Source: CAD feature listing. Evaluate the final solid. Frame: model axes, mm. Face numbers are marked on the shaded views. A direction names the side the tool comes from. Give positions to 0.01 mm unless a question says otherwise; leave off trailing zeros. Loops run counter-clockwise (first coordinate to the right, second up) from the corner with the lowest first, then second, coordinate; pieces in that order, holes last.
from build123d import *

# Parameters (mm, degrees)
F0_R     = 40
F1_DEPTH = 25
F3_R     = 25
F4_DEPTH = 19.775010108
F5_R     = 4.5
F6_DEPTH = 50.0010001


with BuildPart() as f1:
    # F0 (on Front) → F1 (new body, symmetric)
    with BuildSketch(Plane.XZ):
        Circle(F0_R)
    extrude(amount=F1_DEPTH, both=True)

    # F3 (on offset) → F4 (join, up to face)
    with BuildSketch(Plane.YZ.offset(-50)):
        Circle(F3_R)
    extrude(amount=F4_DEPTH)

    # F5 (on face) → F6 (cut, through all)
    with BuildSketch(Plane.XZ.offset(25)):
        Circle(F5_R)
    extrude(amount=-F6_DEPTH, mode=Mode.SUBTRACT)


solid = f1.part
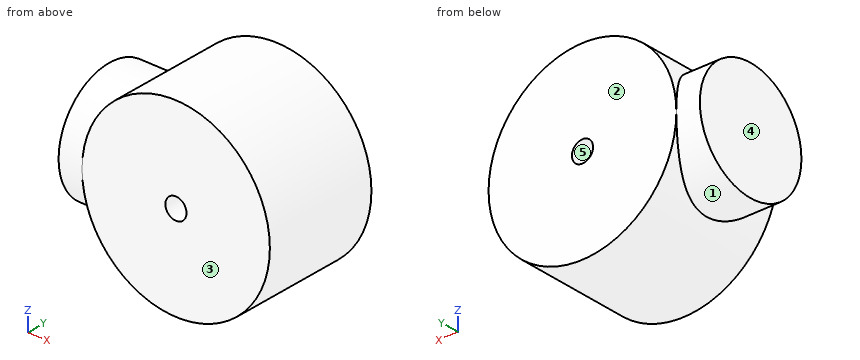
1) Pull-direction query (X, two-part tool) for the marked faces 3, 4 and 5; classes: released by +X, released by -X, zero draft, split by the parting line, or undercut.
Checks:
face 3: zero draft
face 4: released by -X
face 5: undercut
2) Cut plane D-D (x = -18.5). Return loops of the section in (y, z), and give its area (3 significant figures).
Checks:
outline: (-25, -35.46) - (25, -35.46) - (25, 35.46) - (-25, 35.46) - close
area: 3,550 mm2
3) Reachability of the marked faces 1 and 2 from +Z, -Z, +X, -X, +Y, -Y: full face, straight path, thin tool, end or side. Return the list, or none.
Checks:
face 1: -X
face 2: +Z, -Z, +X, -X, +Y
4) Cut plane A-A (x = 0). Return loops of the section in (y, z).
Checks:
outline: (-25, -40) - (25, -40) - (25, -4.5) - (-25, -4.5) - close; (-25, 4.5) - (25, 4.5) - (25, 40) - (-25, 40) - close
5) Ray query, probe 1 along Z at (x, y) = (0, 5); probe 2 along X at (y, z) = (10.5, -2.5); probe 3 along X at (y, z) = (8.5, 3). Return the intervals inside material, ascending.
Checks:
probe 1: z = -40 to -4.5, 4.5 to 40
probe 2: x = -50 to -3.74, 3.74 to 39.92
probe 3: x = -50 to -3.35, 3.35 to 39.89
6) Cut plane C-C (z = 19.5). Return loops of the section in (x, y), and give its area (3 significant figures).
Checks:
outline: (-50, -15.64) - (-34.92, -15.64) - (-34.92, -25) - (34.92, -25) - (34.92, 25) - (-34.92, 25) - (-34.92, 15.64) - (-50, 15.64) - close
area: 3,960 mm2
7) Contact query for flat-ended pins moving along their axis: P1, Ø6, axis at y = -8.5, z = -30, coming from the -X side; P2, Ø1, axis at y = -18, z = 13.5, coming from the +X side; P3, Ø1, axis at x = -12, y = -18.5, coming from the -Z side. Output: stop coordinate, or through.
Checks:
P1: stops at x = -29.51
P2: stops at x = 37.83
P3: stops at z = -38.31
